```python
from build123d import *

# Parameters (mm, degrees)
F0_W           = 50.8
F0_H           = 50.8
F1_DEPTH       = 9.525
F3_D           = 3.96875
F3_DEPTH       = 12.7
F3_TIP         = 1.1923327909
F4_D           = 3
F4_CBORE_D     = 4.7625
F4_CBORE_DEPTH = 3.175
F5_D           = 4.7625
F5_DEPTH       = 12.7
F5_TIP         = 1.4307993491
F6_R           = 20.32
F6_R_2         = 1.5
F6_R_3         = 2.38125
F7_DEPTH       = 4.7625


with BuildPart() as f1:
    # F0 (on Front) → F1 (new body)
    with BuildSketch(Plane.XZ):
        with Locations((25.4, 25.4)):
            Rectangle(F0_W, F0_H)
    extrude(amount=F1_DEPTH)

    # F3
    with Locations(Plane(origin=(0, 0, 0), x_dir=(0, -1, 0), z_dir=(-1, 0, 0))):
        with Locations((4.7625, 44.45), (4.7625, 6.35)):
            Hole(F3_D / 2, depth=F3_DEPTH)
            with Locations((0, 0, -(F3_DEPTH + F3_TIP / 2))):  # 118° drill point
                Cone(0, F3_D / 2, F3_TIP, mode=Mode.SUBTRACT)

    # F4 (through all)
    with Locations(Plane(origin=(0, 0, 0), x_dir=(1, 0, 0), z_dir=(0, 1, 0))):
        with Locations((25.4, -34.9), (15.9, -25.4), (25.4, -15.9), (34.9, -25.4)):
            CounterBoreHole(F4_D / 2, F4_CBORE_D / 2, F4_CBORE_DEPTH)

    # F5
    with Locations(Plane(origin=(0, 0, 0), x_dir=(1, 0, 0), z_dir=(0, 1, 0))):
        with Locations((25.4, -25.4)):
            Hole(F5_D / 2, depth=F5_DEPTH)
            with Locations((0, 0, -(F5_DEPTH + F5_TIP / 2))):  # 118° drill point
                Cone(0, F5_D / 2, F5_TIP, mode=Mode.SUBTRACT)

    # F6 (on face) → F7 (cut)
    with BuildSketch(Plane.XZ.offset(9.525)):
        with Locations((25.4, 25.4)):
            Circle(F6_R)
        with Locations((25.4, 15.9)):
            Circle(F6_R_2, mode=Mode.SUBTRACT)
        with Locations((15.9, 25.4)):
            Circle(F6_R_2, mode=Mode.SUBTRACT)
        with Locations((25.4, 25.4)):
            Circle(F6_R_3, mode=Mode.SUBTRACT)
        with Locations((34.9, 25.4)):
            Circle(F6_R_2, mode=Mode.SUBTRACT)
        with Locations((25.4, 34.9)):
            Circle(F6_R_2, mode=Mode.SUBTRACT)
    extrude(amount=-F7_DEPTH, mode=Mode.SUBTRACT)


solid = f1.part
```
Part model, mm, in its own coordinate system. A direction names the side the tool comes from. Round coordinates to 2 decimals unless told otherwise and drop trailing zeros. Order: outer loops, then holes, each group sorted by start corner. A loop starts at its lowest first (then second) coordinate and runs counter-clockwise, first axis right, second up. Notation, with made-up numbers: M 60.5,37.25 L 66.5,37.25 A5 ccw 66.5,46.25 Z; hole C 10.5,-18 d2. An arc over 180 degrees is marked long. Answer in a Markdown table with one row per item. Add a question column.
Q1. Wall check: L1, parallel to Z at x = 25.4, y = -4.2; L2, parallel to X at y = -1.4, z = 25.4. Give the ranges that are in metal, low to high. Write a range as from..to.
Q2. 3-axis set-ups, long thin cutter, end or side, ignore diameter. For faces 5 (the face through (33.01, -1.57, 26.85)), 6 (the face through (6.44, -2.93, 5.59)), 7 (the face through (25, -4.762, 21)): which of +Z, -Z, +X, -X, +Y, -Y reach the whole face in a straight line?
Q3. Cut at A-A on x = 25.4. Give the cut face in (y, z) (1 decimal).
Q4. Pin check, flat tips, straight feed: pin 1 (7.5 mm diameter, centred on x = 25.4, z = 34.9, fed in from -Y); pin 2 (1.4 mm diameter, centred on x = 24.5, z = 16, fed in from +Y) (3 decimals). Stop position of each tip, or through.
Q5. Cut at C-C on z = 25.4. Give the cut face in (x, y) (1 decimal), and give its area (3 significant figures).
Q6. Mould opens along Z. For faces 1 (the face through (16.4, -3.175, 27)), 2 (the face through (25, -5, 50.8)), 3 (the face through (27, -3.175, 35.4)), 4 (the face through (31, 0, 26)) say: +Z half, -Z half, draft (parallel to the pull), parting line (faces both ways), or undercut.
Q7. Cut at B-B on y = -1.25. Give the cut face in (x, z).
Q8. Cut at D-D on x = 15.9. Give the cut face in (y, z) (1 decimal), and give its area (3 significant figures).
Established:
| question | item | result |
|---|---|---|
| 1 | L1 | z = 0..14.4, 17.4..23.02, 27.78..33.4, 36.4..50.8 |
| 1 | L2 | x = 0..13.52, 18.28..23.02, 27.78..32.52, 37.28..50.8 |
| 2 | face 5 | +Y |
| 2 | face 6 | -X |
| 2 | face 7 | -Y |
| 3 | outline | M -9.5,0 L 0,0 L 0,13.5 L -3.2,13.5 L -3.2,14.4 L -4.8,14.4 L -4.8,5.1 L -9.5,5.1 Z; M -9.5,45.7 L -4.8,45.7 L -4.8,36.4 L -3.2,36.4 L -3.2,37.3 L 0,37.3 L 0,50.8 L -9.5,50.8 Z; M -4.8,17.4 L -3.2,17.4 L -3.2,18.3 L 0,18.3 L 0,23 L -4.8,23 Z; M -4.8,27.8 L 0,27.8 L 0,32.5 L -3.2,32.5 L -3.2,33.4 L -4.8,33.4 Z |
| 4 | pin 1 | stops at y = -4.76 |
| 4 | pin 2 | stops at y = -3.175 |
| 5 | outline | M 0,-9.5 L 5.1,-9.5 L 5.1,-4.8 L 14.4,-4.8 L 14.4,-3.2 L 13.5,-3.2 L 13.5,0 L 0,0 Z; M 17.4,-4.8 L 23,-4.8 L 23,0 L 18.3,0 L 18.3,-3.2 L 17.4,-3.2 Z; M 27.8,-4.8 L 33.4,-4.8 L 33.4,-3.2 L 32.5,-3.2 L 32.5,0 L 27.8,0 Z; M 36.4,-4.8 L 45.7,-4.8 L 45.7,-9.5 L 50.8,-9.5 L 50.8,0 L 37.3,0 L 37.3,-3.2 L 36.4,-3.2 Z |
| 5 | area | 228 mm2 |
| 6 | face 1 | undercut |
| 6 | face 2 | +Z half |
| 6 | face 3 | undercut |
| 6 | face 4 | draft |
| 7 | outline | M 0,0 L 50.8,0 L 50.8,50.8 L 0,50.8 Z; hole C 15.9,25.4 d4.76; hole C 25.4,15.9 d4.76; hole C 25.4,25.4 d4.76; hole C 25.4,34.9 d4.76; hole C 34.9,25.4 d4.76 |
| 8 | outline | M -9.5,0 L 0,0 L 0,23 L -3.2,23 L -3.2,23.9 L -4.8,23.9 L -4.8,7.4 L -9.5,7.4 Z; M -9.5,43.4 L -4.8,43.4 L -4.8,26.9 L -3.2,26.9 L -3.2,27.8 L 0,27.8 L 0,50.8 L -9.5,50.8 Z |
| 8 | area | 293 mm2 |
